Check sheet for the modelled part. Datum: model origin and axes. Units: mm. A direction names the side the tool comes from. Round coordinates to 2 decimals unless told otherwise and drop trailing zeros. Use CSV: the item, a comma, the result in double quotes.
```python
from build123d import *

# Parameters (mm, degrees)
SKETCH_1_R          = 110
EXTRUDE_1_DEPTH     = 14
SKETCH_2_R          = 85
EXTRUDE_2_DEPTH     = 7
SKETCH_3_R          = 55
CUT_EXTRUDE_1_DEPTH = 157.974520225
FILLET_1_R          = 7
SKETCH_5_R          = 5.5
CUT_EXTRUDE_2_DEPTH = 157.974520225
SKETCH_6_R          = 5.5
CUT_EXTRUDE_3_DEPTH = 157.974520225
SKETCH_7_R          = 67.5
CUT_EXTRUDE_4_DEPTH = 5
SKETCH_8_R          = 9
CUT_EXTRUDE_5_DEPTH = 11
SKETCH_10_R         = 4
CUT_EXTRUDE_6_DEPTH = 157.974520225


with BuildPart() as part:
    # 草图1 → 拉伸1 (new body)
    with BuildSketch(Plane.XY):
        Circle(SKETCH_1_R)
    extrude(amount=EXTRUDE_1_DEPTH)

    # 草图2 → 拉伸2 (add)
    with BuildSketch(Plane.XY.offset(14)):
        Circle(SKETCH_2_R)
    extrude(amount=EXTRUDE_2_DEPTH)

    # 草图3 → 切除-拉伸1 (cut, through all)
    with BuildSketch(Plane(origin=(0, 0, 0), x_dir=(-1, 0, 0), z_dir=(0, 0, -1))):
        Circle(SKETCH_3_R)
    extrude(amount=-CUT_EXTRUDE_1_DEPTH, mode=Mode.SUBTRACT)

    # 圆角1
    fillet_1_edges = [part.edges().sort_by_distance(p)[0] for p in [
        (-110, 0, 0),
    ]]
    fillet(fillet_1_edges, radius=FILLET_1_R)

    # 草图5 → 切除-拉伸2 (cut, through all)
    with BuildSketch(Plane(origin=(0, 0, 0), x_dir=(-1, 0, 0), z_dir=(0, 0, -1))):
        with Locations((0, 95)):
            Circle(SKETCH_5_R)
        with Locations((67.175144213, 67.175144213)):
            Circle(SKETCH_5_R)
        with Locations((95, 0)):
            Circle(SKETCH_5_R)
        with Locations((67.175144213, -67.175144213)):
            Circle(SKETCH_5_R)
        with Locations((0, -95)):
            Circle(SKETCH_5_R)
        with Locations((-67.175144213, -67.175144213)):
            Circle(SKETCH_5_R)
        with Locations((-95, 0)):
            Circle(SKETCH_5_R)
        with Locations((-67.175144213, 67.175144213)):
            Circle(SKETCH_5_R)
    extrude(amount=-CUT_EXTRUDE_2_DEPTH, mode=Mode.SUBTRACT)

    # 草图6 → 切除-拉伸3 (cut, through all)
    with BuildSketch(Plane(origin=(0, 0, 0), x_dir=(-1, 0, 0), z_dir=(0, 0, -1))):
        with Locations((0, 75)):
            Circle(SKETCH_6_R)
        with Locations((64.951905284, 37.5)):
            Circle(SKETCH_6_R)
        with Locations((64.951905284, -37.5)):
            Circle(SKETCH_6_R)
        with Locations((0, -75)):
            Circle(SKETCH_6_R)
        with Locations((-64.951905284, -37.5)):
            Circle(SKETCH_6_R)
        with Locations((-64.951905284, 37.5)):
            Circle(SKETCH_6_R)
    extrude(amount=-CUT_EXTRUDE_3_DEPTH, mode=Mode.SUBTRACT)

    # 草图7 → 切除-拉伸4 (cut)
    with BuildSketch(Plane.XY.offset(21)):
        Circle(SKETCH_7_R)
    extrude(amount=-CUT_EXTRUDE_4_DEPTH, mode=Mode.SUBTRACT)

    # 草图8 → 切除-拉伸5 (cut)
    with BuildSketch(Plane(origin=(0, 0, 0), x_dir=(-1, 0, 0), z_dir=(0, 0, -1))):
        with Locations((0, 75)):
            Circle(SKETCH_8_R)
        with Locations((64.951905284, 37.5)):
            Circle(SKETCH_8_R)
        with Locations((64.951905284, -37.5)):
            Circle(SKETCH_8_R)
        with Locations((0, -75)):
            Circle(SKETCH_8_R)
        with Locations((-64.951905284, -37.5)):
            Circle(SKETCH_8_R)
        with Locations((-64.951905284, 37.5)):
            Circle(SKETCH_8_R)
    extrude(amount=-CUT_EXTRUDE_5_DEPTH, mode=Mode.SUBTRACT)

    # 草图10 → 切除-拉伸6 (cut, through all)
    with BuildSketch(Plane(origin=(0, 0, 0), x_dir=(-1, 0, 0), z_dir=(0, 0, -1))):
        with Locations((18.76438077, 70.029622406)):
            Circle(SKETCH_10_R)
        with Locations((70.029622406, -18.76438077)):
            Circle(SKETCH_10_R)
        with Locations((-18.76438077, -70.029622406)):
            Circle(SKETCH_10_R)
        with Locations((-70.029622406, 18.76438077)):
            Circle(SKETCH_10_R)
    extrude(amount=-CUT_EXTRUDE_6_DEPTH, mode=Mode.SUBTRACT)


solid = part.part
```
Q1. Scan lines: L1, parallel to Y at x = 0, z = 19.25; L2, parallel to X at y = -65, z = 9.5; L3, parallel to X at y = -36.5, z = 8. Record each from-to range of solid material in increasing order.
Result sheet:
L1,"y = -85 to -80.5, -69.5 to -67.5, 67.5 to 69.5, 80.5 to 85"
L2,"x = -88.74 to -72.23, -62.12 to 62.12, 72.23 to 88.74"
L3,"x = -103.77 to -73.9, -56.01 to -41.14, 41.14 to 56.01, 73.9 to 103.77"
Q2. Sectioned sample at A-A, the plane z = 2.5. State how many separate pieces and enclosed holes the cut face has, then the cut area to 3 significant figures.
Result sheet:
separate pieces,"1"
enclosed holes,"19"
area,"24,900 mm^2"
Q3. Go/stop test with flat-tipped pins: pin 1 (20.5 mm diameter, centred on x = -64.95, y = -37.5, fed in from +Z); pin 2 (4 mm diameter, centred on x = -49, z = 12.5, fed in from -Y); pin 3 (10 mm diameter, centred on y = 72, z = 11, fed in from -X); pin 4 (9 mm diameter, centred on x = 0, y = 95, fed in from -Z). Record where each tip stops, or that it passes through.
Result sheet:
pin 1,"stops at z = 21"
pin 2,"stops at y = -99.45"
pin 3,"stops at x = -87.24"
pin 4,"passes through"
Q4. Mould release check, pull along X, two halves, no side actions. Record for faces 1 (the face through (-67.453, -51.721, 17.451)), 2 (the face through (-70.2, -35.85, 15.93)): pulls with the +X half, pulls with the -X half, needs draft (parallel to the pull), parting line crosses it, or undercut.
Result sheet:
face 1,"parting line crosses it"
face 2,"undercut"
Q5. Access from +Z, -Z, +X, -X, +Y, -Y to the whole of each face (thin tool, end or side, straight path). Record for faces 3 (the face through (-4, -71, 11)), 4 (the face through (0.716, 80.453, 15.93)).
Result sheet:
face 3,"-Z"
face 4,"+Z, -Z"
